The listing builds one solid part. Answer for the finished solid, in the listing's coordinates (mm). A direction names the side the tool comes from. Coordinates: 2 decimals unless noted, no trailing zeros. Loops run counter-clockwise (first coordinate to the right, second up) from the corner with the lowest first, then second, coordinate; pieces in that order, holes last. Notation, with made-up numbers: (-30.75, -4) - (25.25, -4) arc R10 cw to (25.25, 12) - close; hole circle Ø1 at (84, -15.75). An arc over 180 degrees is marked (long way). Put each result on its own line as item: value.
Autodesk Inventor part; units mm, degrees
ref_plane "YZ Plane" through (0, 0, 0) normal (1, 0, 0) x (0, 1, 0)
ref_plane "XZ Plane" through (0, 0, 0) normal (0, 1, 0) x (-1, 0, 0)
ref_plane "XY Plane" through (0, 0, 0) normal (0, 0, 1) x (1, 0, 0)
sketch "Sketch1" plane through (0, 0, 0) normal (0, 0, 1) x (1, 0, 0)
  circle A0 centre (0, 0) radius 57.5
  line L0 (-57.5, 0) -> (57.5, 0)
  circle A1 centre (0, 0) radius 55
  point P0 (55, 0)
  point P1 (-55, 0)
  dimension "d0" = 115
  dimension "d2" = 110
extrude "Extrusion1" add sketch "Sketch1" along normal mid plane 620 contours L0 A1 A0 | A0 L0 A1
sketch "Sketch3" plane through (0, 0, 310) normal (0, 0, 1) x (1, 0, 0)
  circle A0 centre (0, 0) radius 57.5
  dimension "d5" = 115
extrude "Extrusion2" add sketch "Sketch3" along normal blind 3
sketch "Sketch4" plane through (0, 0, -310) normal (0, 0, -1) x (-1, 0, 0)
  circle A0 centre (0, 0) radius 57.5
  dimension "d8" = 115
extrude "Extrusion3" add sketch "Sketch4" along normal blind 3
sketch "Sketch5" plane through (0, 0, 0) normal (0, 1, 0) x (-1, 0, 0)
  line L0 (0, 0) -> (0, 270) construction
  line L1 (45, 310) -> (-45, 310)
  line L2 (-45, 310) -> (-45, 230)
  line L3 (-45, 230) -> (45, 230)
  line L4 (45, 230) -> (45, 310)
  line L5 (45, 310) -> (-45, 230) construction
  line L6 (-45, 310) -> (45, 230) construction
  line L7 (0, 0) -> (20, 0) construction
  line L8 (0, 0) -> (0, -295)
  line L9 (-45, -280) -> (45, -280)
  line L10 (45, -280) -> (45, -310)
  line L11 (45, -310) -> (-45, -310)
  line L12 (-45, -310) -> (-45, -280)
  line L13 (-45, -280) -> (45, -310) construction
  line L14 (45, -280) -> (-45, -310) construction
  dimension "d11" = 270
  dimension "d12" = 90
  dimension "d13" = 80
  dimension "d14" = 20
  dimension "d37" = 295
  dimension "d38" = 90
  dimension "d39" = 30
extrude "Extrusion4" cut sketch "Sketch5" against normal blind 80
sketch "Sketch6" plane through (0, 0, 0) normal (0, 1, 0) x (-1, 0, 0)
  line L0 (60, 135) -> (-60, 135)
  line L1 (-60, 135) -> (-60, -135)
  line L2 (-60, -135) -> (60, -135)
  line L3 (60, -135) -> (60, 135)
  line L4 (60, 135) -> (-60, -135) construction
  line L5 (-60, 135) -> (60, -135) construction
  point P0 (0, 0)
  dimension "d17" = 120
  dimension "d18" = 270
extrude "Extrusion5" cut sketch "Sketch6" along normal blind 100
sketch "Sketch7" plane through (0, 0, 0) normal (1, 0, 0) x (0, 1, 0)
  line L0 (6, 280) -> (-6, 280)
  line L1 (-6, 280) -> (-6, -280)
  line L2 (-6, -280) -> (6, -280)
  line L3 (6, -280) -> (6, 280)
  line L4 (6, 280) -> (-6, -280) construction
  line L5 (-6, 280) -> (6, -280) construction
  line L6 (-6, 0) -> (6, 0)
  line L7 (6, 0) -> (-6, 0)
  line L8 (-6, 0) -> (-6, -290)
  line L9 (-6, -290) -> (6, -290)
  line L10 (6, -290) -> (6, 0)
  line L11 (6, 0) -> (-6, 0)
  line L12 (-6, 0) -> (-6, 260)
  line L13 (-6, 260) -> (6, 260)
  line L14 (6, 260) -> (6, 0)
  point P0 (0, 0)
  point P1 (6, 260)
  point P2 (-6, 260)
  dimension "d21" = 12
  dimension "d22" = 560
  dimension "d34" = 290
  dimension "d35" = 12
  dimension "d36" = 260
extrude "Extrusion6" cut sketch "Sketch7" along normal mid plane 200 contours L3 L6 L1 L13 | L3 L2 L1 L6 | L10 L9 L8 L2
sketch "Sketch8" plane through (0, 0, 313) normal (0, 0, 1) x (1, 0, 0)
  circle A0 centre (0, 0) radius 15
  dimension "d25" = 30
extrude "Extrusion7" cut sketch "Sketch8" against normal blind 1000
properties part number "GUIA_DE_OBJETO"
1) For a pull along Y with two mould halves and no side action, classify faces 1 (the face through (47.793, -31.97, 4.382)), 2 (the face through (-8, 55, -135)), 3 (the face through (-14.985, 0.66, -311.479)) as pulls with the +Y half, pulls with the -Y half, needs draft (parallel to the pull), parting line crosses it, or undercut.
Found:
face 1: parting line crosses it
face 2: needs draft
face 3: undercut
2) For faces 4 (the face through (12, -12, 313)), 5 (the face through (29.568, -46.376, -4.34)), 6 (the face through (8, 55, 135)), determine the directions among +Z, -Z, +X, -X, +Y, -Y from which every point of the face is accessible in a straight line to the end or side of a thin tool.
Found:
face 4: +Z, +X, -X, +Y, -Y
face 5: none
face 6: +X, -X, +Y
3) The part is cut by section A-A (y = 0). Give the vertices of the cut face in (x, z).
Found:
outline: (-57.5, -313) - (-15, -313) - (-15, -310) - (-55, -310) - (-55, -290) - (-57.5, -290) - close; (-57.5, 260) - (-55, 260) - (-55, 310) - (-15, 310) - (-15, 313) - (-57.5, 313) - close; (15, -313) - (57.5, -313) - (57.5, -290) - (55, -290) - (55, -310) - (15, -310) - close; (15, 310) - (55, 310) - (55, 260) - (57.5, 260) - (57.5, 313) - (15, 313) - close
4) Straight lines are drawn through the part: L1, parallel to Z at x = -33, y = -23.5; L2, parallel to Y at x = 0, z = 311.7; L3, parallel to Y at x = -39, z = 214.5. For each, find the intervals that lie inside material, in ascending order. Write a range as [from, to].
Found:
L1: z = [-313, -310], [310, 313]
L2: y = [-57.5, -15], [15, 57.5]
L3: y = [-42.25, -38.78], [38.78, 42.25]
5) The part is cut by section B-B (x = 0). Give the vertices of the cut face in (y, z).
Found:
outline: (-57.5, -313) - (-15, -313) - (-15, -310) - (-57.5, -310) - close; (-57.5, -280) - (-55, -280) - (-55, 230) - (-57.5, 230) - close; (-57.5, 310) - (-15, 310) - (-15, 313) - (-57.5, 313) - close; (15, -313) - (57.5, -313) - (57.5, -135) - (55, -135) - (55, -310) - (15, -310) - close; (15, 310) - (55, 310) - (55, 135) - (57.5, 135) - (57.5, 313) - (15, 313) - close
6) The part is cut by section D-D (y = 38). Give the vertices of the cut face in (x, z).
Found:
outline: (-43.15, -313) - (43.15, -313) - (43.15, -135) - (39.76, -135) - (39.76, -310) - (-39.76, -310) - (-39.76, -135) - (-43.15, -135) - close; (-43.15, 135) - (-39.76, 135) - (-39.76, 310) - (39.76, 310) - (39.76, 135) - (43.15, 135) - (43.15, 313) - (-43.15, 313) - close
7) Each of these flat-tipped pins is pushed along its axis until it touches: pin 1 (12 mm diameter, centred on x = -22.5, z = 192.5, fed in from -Y); pin 2 (10 mm diameter, centred on x = 40.5, z = 133, fed in from -Y); pin 3 (2 mm diameter, centred on y = -34.5, z = -289.5, fed in from -X); pin 4 (18 mm diameter, centred on x = 0, y = 0, fed in from -Z). Where does it stop, or does it pass through?
Found:
pin 1: stops at y = -55.08
pin 2: stops at y = -45.23
pin 3: stops at x = -46.73
pin 4: passes through
